The listing builds one solid part. Answer for the finished solid, in the listing's coordinates (mm). A direction names the side the tool comes from. Round coordinates to 2 decimals unless told otherwise and drop trailing zeros. Loops run counter-clockwise (first coordinate to the right, second up) from the corner with the lowest first, then second, coordinate; pieces in that order, holes last. Notation, with made-up numbers: M 72,75.5 L 81,75.5 A22 cw 81,93.5 Z; hole C 1,39 d4. An arc over 180 degrees is marked long. Put each result on its own line as item: value. Start each with the question number.
(1) Flat-ended cylindrical pins translate along their axes: P1, Ø5, axis at y = 33.5, z = 119, coming from the -X side; P2, Ø8, axis at x = 37, z = 52.5, coming from the +Y side; P3, Ø0.5, axis at x = -56.5, y = 1.5, coming from the +Z side. Find the tip coordinate at first contact, or state that the pin passes through.
(2) Section A-A, the plane z = 100 is taken. Determine the outline of the cut face in (x, y), then the cut area to 3 significant figures.
(3) Section C-C, the plane y = -47 is taken. Determine the outline of the cut face in (x, z).
(4) Determine the mould class of faces 1 (the face through (-57.095, 2.513, 112.7)), 2 (the face through (-1, 1, 0.8)), 3 (the face through (40, 40, 228.6)) for opening direction X: released by +X, released by -X, zero draft, split by the parting line, or undercut.
(5) Which of the six approach directions +Z, -Z, +X, -X, +Y, -Y give full straight-line access (tool end or side, diameter ignored) to faces 4 (the face through (-46, 33, 228.6)), 5 (the face through (53.748, 16.926, 113.105))?
(6) Section B-B, the plane x = -50 is taken. Determine the outline of the cut face in (y, z).
(7) Straight lines are drawn through the part: line 1 (Y direction, x = 4, z = 35); line 2 (Y direction, x = 0, z = 127.5). For each, find the intervals that lie inside material, in ascending order.
```python
from build123d import *

# Parameters (mm, degrees)
F0_R          = 57.15
F1_DEPTH      = 228.6
F2_T          = -0.8
F3_R          = 1
F4_DEPTH      = 0.8
F5_W          = 8
F5_H          = 2
F6_DEPTH      = 57.151
F6_DEPTH_BACK = 57.151
F7_W          = 8
F7_H          = 4
F8_DEPTH      = 57.151
F8_DEPTH_BACK = 57.151


with BuildPart() as f1:
    # F0 (on Top) → F1 (new body)
    with BuildSketch(Plane.XY):
        Circle(F0_R)
    extrude(amount=F1_DEPTH)

    # F2
    f2_openings = [f1.faces().sort_by_distance(p)[0] for p in [
        (0, 0, 228.6),
    ]]
    offset(amount=F2_T, openings=f2_openings)

    # F3 (on face) → F4 (cut, through all)
    with BuildSketch(Plane.XY.offset(0.8)):
        Circle(F3_R)
    extrude(amount=-F4_DEPTH, mode=Mode.SUBTRACT)

    # F5 (on Front) → F6 (cut, two sides)
    with BuildSketch(Plane.XZ) as f6_sk:
        with Locations((0, 227.6)):
            Rectangle(F5_W, F5_H)
    extrude(amount=-F6_DEPTH, mode=Mode.SUBTRACT)
    extrude(f6_sk.sketch, amount=F6_DEPTH_BACK, mode=Mode.SUBTRACT)

    # F7 (on Right) → F8 (cut, two sides)
    with BuildSketch(Plane.YZ) as f8_sk:
        with Locations((0, 226.6)):
            Rectangle(F7_W, F7_H)
    extrude(amount=-F8_DEPTH, mode=Mode.SUBTRACT)
    extrude(f8_sk.sketch, amount=F8_DEPTH_BACK, mode=Mode.SUBTRACT)


solid = f1.part
```
Recorded:
1. P1: stops at x = -48.01
1. P2: stops at y = 46.66
1. P3: stops at z = 224.6
2. outline: C 0,0 d114.3; hole C 0,0 d112.7
2. area: 285 mm²
3. outline: M -32.51,0 L 32.51,0 L 32.51,228.6 L 31.09,228.6 L 31.09,0.8 L -31.09,0.8 L -31.09,228.6 L -32.51,228.6 Z
4. face 1: split by the parting line
4. face 2: undercut
4. face 3: zero draft
5. face 4: +Z, +X, -X, +Y, -Y
5. face 5: +Z
6. outline: M -27.68,0 L 27.68,0 L 27.68,228.6 L 25.99,228.6 L 25.99,0.8 L -25.99,0.8 L -25.99,228.6 L -27.68,228.6 Z
7. line 1: y = -57.01 to -56.21, 56.21 to 57.01
7. line 2: y = -57.15 to -56.35, 56.35 to 57.15
